Can you work these out from the model? Positions are in its coordinate system, mm. A direction names the side the tool comes from. Coordinates: 2 decimals unless noted, no trailing zeros. Order: outer loops, then holes, each group sorted by start corner. A loop starts at its lowest first (then second) coordinate and runs counter-clockwise, first axis right, second up. Notation, with made-up numbers: (76.25, -12.75) -> (87.25, -12.75) arc R28 ccw to (87.25, 16.25) -> close; hole circle Ø8 at (53.5, 57). An arc over 180 degrees is marked (long way). Return JSON: item names as keys, results as strings. Group by question number.
1) For faces 5 (the flat face through (-65.9, 127, 0.4)), 6 (the flat face through (-15, 7.4, -1.9)), 7 (the flat face through (-7, 12, -6)), which set-ups out of +Z, -Z, +X, -X, +Y, -Y let a thin tool reach every point of the face, with its end or its side?
2) If I drill on probe 1 along Y at (x, z) = (-124.5, -6); probe 2 along Z at (x, y) = (-99.5, 72), over which ranges is the centre line in solid material (lowest first)? Write a range as from..to.
3) For pin 1 (5 mm diameter, centred on x = -85, y = 101.5, fed in from -Z), with a flat end and sliding along its axis, tell me the tip position at first contact or that it passes through.
4) Thinking about a two-plate mould opening in Z: for faces 1 (the cylindrical face through (-122.395, 2.095, -5.133)), 2 (the cylindrical face through (-7.395, 2.095, -5.133)), 3 (the flat face through (-7, 121, -12)), 4 (the flat face through (-122, 115, -6)), which applies, +Z half, -Z half, draft (parallel to the pull), parting line (faces both ways), or undercut?
5) If we section it at A-A, the plane y = 121: Please give me the cut outline in (x, z).
6) If we section it at D-D, the plane x = -17: Please give me the cut outline in (y, z).
7) If we section it at B-B, the plane z = -6: State how many separate pieces and enclosed holes the cut face has, then the cut area to 3 significant figures.
8) If we section it at C-C, the plane x = -120: Please give me the cut outline in (y, z), then the cut area to 3 significant figures.
from build123d import *

# Parameters (mm, degrees)
ESQUISSE1_W             = 130
ESQUISSE1_H             = 127
BOSS_EXTRU_1_DEPTH      = 3
ESQUISSE2_W             = 12
ESQUISSE2_H             = 12
ESQUISSE2_R             = 4
BOSS_EXTRU_2_DEPTH      = 130
ESQUISSE3_W             = 100
ESQUISSE3_H             = 12
ENL_V_MAT_EXTRU_1_DEPTH = 160


with BuildPart() as part:
    # Esquisse1 → Boss.-Extru.1 (new body)
    with BuildSketch(Plane.XY):
        with Locations((-65, 63.5)):
            Rectangle(ESQUISSE1_W, ESQUISSE1_H)
    extrude(amount=BOSS_EXTRU_1_DEPTH)

    # Esquisse2 → Boss.-Extru.2 (add)
    with BuildSketch(Plane(origin=(0, 0, 0), x_dir=(0, 0, -1), z_dir=(1, 0, 0))):
        with Locations((6, 6)):
            Rectangle(ESQUISSE2_W, ESQUISSE2_H)
        with Locations((6, 6)):
            Circle(ESQUISSE2_R, mode=Mode.SUBTRACT)
        with Locations((6, 121)):
            Rectangle(ESQUISSE2_W, ESQUISSE2_H)
        with Locations((6, 121)):
            Circle(ESQUISSE2_R, mode=Mode.SUBTRACT)
    extrude(amount=-BOSS_EXTRU_2_DEPTH)

    # Esquisse3 → Enlèv. mat.-Extru.1 (cut)
    with BuildSketch(Plane(origin=(0, 127, 0), x_dir=(1, 0, 0), z_dir=(0, 1, 0))):
        with Locations((-65, 6)):
            Rectangle(ESQUISSE3_W, ESQUISSE3_H)
    extrude(amount=-ENL_V_MAT_EXTRU_1_DEPTH, mode=Mode.SUBTRACT)


solid = part.part
Result sheet:
{
 "1": {"face 5": "+Z, -Z, +X, -X, +Y", "face 6": "-Z, +Y, -Y", "face 7": "-Z, +X, -X"},
 "2": {"probe 1": "y = 0..2, 10..12, 115..117, 125..127", "probe 2": "z = 0..3"},
 "3": {"pin 1": "stops at z = 0"},
 "4": {"face 1": "undercut", "face 2": "undercut", "face 3": "-Z half", "face 4": "draft"},
 "5": {"outline": "(-130, -12) -> (-115, -12) -> (-115, -10) -> (-130, -10) -> close; (-130, -2) -> (-115, -2) -> (-115, 0) -> (-15, 0) -> (-15, -2) -> (0, -2) -> (0, 3) -> (-130, 3) -> close; (-15, -12) -> (0, -12) -> (0, -10) -> (-15, -10) -> close"},
 "6": {"outline": "(0, 0) -> (127, 0) -> (127, 3) -> (0, 3) -> close"},
 "7": {"separate pieces": "8", "enclosed holes": "0", "area": "240 mm2"},
 "8": {"outline": "(0, -12) -> (12, -12) -> (12, 0) -> (115, 0) -> (115, -12) -> (127, -12) -> (127, 3) -> (0, 3) -> close; hole circle Ø8 at (6, -6); hole circle Ø8 at (121, -6)", "area": "568 mm2"}
}
